Build history of the part. All positions in model axes, mm. A direction names the side the tool comes from. Give positions to 0.01 mm unless a question says otherwise; leave off trailing zeros. Write each loop counter-clockwise with the first axis right and the second up, starting at its lowest first coordinate (ties: lowest second). Pieces come first, ordered by that corner, then holes. Notation, with made-up numbers: (-31.75, 30.25) -> (11.25, 30.25) arc R21 cw to (11.25, 61.25) -> close; hole circle Ø10 at (88.5, 65). An arc over 180 degrees is marked (long way). Write item = value, one per line. Start each with the question number.
Q1. Drop flat-ended pins along their axis: P1, Ø10.5, axis at y = 13.5, z = 8.5, coming from the -X side; P2, Ø10, axis at y = 24, z = 2, coming from the +X side. Give the stop position or say it passes through.
Q2. Tool access for faces 1 (the face through (-23.14, 2.64, 2.87)), 2 (the face through (0, 38.6, 0)), 3 (the face through (19.11, -10.74, 2.38)): list every direction of +Z, -Z, +X, -X, +Y, -Y with a clear straight run to the whole face (end or side of a thin tool).
Q3. Saw through at A-A, the plane z = 0. List the corners of the cut face in (x, y), then the cut area to 3 significant figures.
Q4. Saw through at C-C, the plane x = 22.5. List the corners of the cut face in (y, z), then the cut area to 3 significant figures.
Q5. Wall check: line 1 (X direction, y = 8, z = 10.5); line 2 (X direction, y = -9, z = -2.5); line 3 (Y direction, x = -18, z = -3). Give the ranges that are in metal, low to high.
Q6. Saw through at B-B, the plane y = 0. List the corners of the cut face in (x, z), then the cut area to 3 significant figures.
Q7. Saw through at D-D, the plane y = 10. List the corners of the cut face in (x, z).
from build123d import *

# Parameters (mm, degrees)
SKETCH2_W           = 35.5
SKETCH2_H           = 35.6
BOSS_EXTRUDE1_DEPTH = 50.6
SKETCH3_R           = 11
BOSS_EXTRUDE2_DEPTH = 2.75
SKETCH4_R           = 3.9
BOSS_EXTRUDE3_DEPTH = 5.35


with BuildPart() as part:
    # Sketch2 → Boss-Extrude1 (new body)
    with BuildSketch(Plane(origin=(0, -12, 0), x_dir=(-1, 0, 0), z_dir=(0, 1, 0))):
        Rectangle(SKETCH2_W, SKETCH2_H)
    extrude(amount=BOSS_EXTRUDE1_DEPTH)

    # Sketch3 → Boss-Extrude2 (add)
    with BuildSketch(Plane(origin=(17.75, 0, 0), x_dir=(0, 0, -1), z_dir=(1, 0, 0))):
        Circle(SKETCH3_R)
    boss_extrude2 = extrude(amount=BOSS_EXTRUDE2_DEPTH)

    # Sketch4 → Boss-Extrude3 (add)
    with BuildSketch(Plane(origin=(20.5, 0, 0), x_dir=(0, 0, -1), z_dir=(1, 0, 0))):
        Circle(SKETCH4_R)
    boss_extrude3 = extrude(amount=BOSS_EXTRUDE3_DEPTH)

    # Mirror1: Boss-Extrude2, Boss-Extrude3 across plane
    add(boss_extrude2.mirror(Plane(origin=(0, 0, 0), x_dir=(0, 0, 1), z_dir=(1, 0, 0))))
    add(boss_extrude3.mirror(Plane(origin=(0, 0, 0), x_dir=(0, 0, 1), z_dir=(1, 0, 0))))


solid = part.part
Report:
q1.P1 = -20.5
q1.P2 = 17.75
q2.face_1 = -X
q2.face_2 = +Z, -Z, +X, -X, +Y
q2.face_3 = +X
q3.outline = (-25.85, -3.9) -> (-20.5, -3.9) -> (-20.5, -11) -> (-17.75, -11) -> (-17.75, -12) -> (17.75, -12) -> (17.75, -11) -> (20.5, -11) -> (20.5, -3.9) -> (25.85, -3.9) -> (25.85, 3.9) -> (20.5, 3.9) -> (20.5, 11) -> (17.75, 11) -> (17.75, 38.6) -> (-17.75, 38.6) -> (-17.75, 11) -> (-20.5, 11) -> (-20.5, 3.9) -> (-25.85, 3.9) -> close
q3.area = 2,000 mm2
q4.outline = circle Ø7.8 at (0, 0)
q4.area = 47.8 mm2
q5.line_1 = -17.75 to 17.75
q5.line_2 = -20.5 to 20.5
q5.line_3 = -10.58 to 10.58
q6.outline = (-25.85, -3.9) -> (-20.5, -3.9) -> (-20.5, -11) -> (-17.75, -11) -> (-17.75, -17.8) -> (17.75, -17.8) -> (17.75, -11) -> (20.5, -11) -> (20.5, -3.9) -> (25.85, -3.9) -> (25.85, 3.9) -> (20.5, 3.9) -> (20.5, 11) -> (17.75, 11) -> (17.75, 17.8) -> (-17.75, 17.8) -> (-17.75, 11) -> (-20.5, 11) -> (-20.5, 3.9) -> (-25.85, 3.9) -> close
q6.area = 1,470 mm2
q7.outline = (-20.5, -4.58) -> (-17.75, -4.58) -> (-17.75, -17.8) -> (17.75, -17.8) -> (17.75, -4.58) -> (20.5, -4.58) -> (20.5, 4.58) -> (17.75, 4.58) -> (17.75, 17.8) -> (-17.75, 17.8) -> (-17.75, 4.58) -> (-20.5, 4.58) -> close
